```python
from build123d import *

# Parameters (mm, degrees)
F0_W     = 2140
F0_H     = 500
F1_DEPTH = 40
F2_W     = 600
F2_H     = 300
F3_DEPTH = 120
F5_D     = 45
F6_W     = 540
F6_H     = 240
F7_DEPTH = 120
F8_R     = 10
F10_D    = 45


with BuildPart() as f1:
    # F0 (on Top) → F1 (new body)
    with BuildSketch(Plane.XY):
        Rectangle(F0_W, F0_H)
    extrude(amount=F1_DEPTH)

    # F2 (on face) → F3 (join)
    with BuildSketch(Plane(origin=(0, 0, 0), x_dir=(1, 0, 0), z_dir=(0, 0, -1))):
        with Locations((-520, 0)):
            Rectangle(F2_W, F2_H)
    extrude(amount=F3_DEPTH)

    # F5 (through all)
    with Locations(Plane(origin=(0, 0, 0), x_dir=(1, 0, 0), z_dir=(0, 0, -1))):
        with Locations((-520, -200)):
            Hole(F5_D / 2)

    # F6 (on face) → F7 (cut)
    with BuildSketch(Plane.XY.offset(40)):
        with Locations((-520, 0)):
            Rectangle(F6_W, F6_H)
    extrude(amount=-F7_DEPTH, mode=Mode.SUBTRACT)

    # F8
    f8_edges = [f1.edges().sort_by_distance(p)[0] for p in [
        (-250, -120, -20),
        (-250, 0, -80),
        (-520, -120, -80),
        (-790, -120, -20),
        (-790, 0, -80),
        (-520, 120, -80),
        (-250, 120, -20),
        (-790, 120, -20),
    ]]
    fillet(f8_edges, radius=F8_R)

    # F10 (through all)
    with Locations(Plane.XY.offset(-80)):
        with Locations((-520, 0)):
            Hole(F10_D / 2)


solid = f1.part
```
Source: CAD feature listing. Evaluate the final solid. Frame: model axes, mm. A direction names the side the tool comes from. Give positions to 0.01 mm unless a question says otherwise; leave off trailing zeros. Order: outer loops, then holes, each group sorted by start corner. A loop starts at its lowest first (then second) coordinate and runs counter-clockwise, first axis right, second up. Notation, with made-up numbers: (-6.75, -20.5) -> (9.25, -20.5) arc R25 ccw to (9.25, 11.5) -> close; hole circle Ø5 at (-23, 48.25). An arc over 180 degrees is marked (long way). Use a Markdown table: item, result.
Q1. Section B-B (y = 0). Return the cut outline in (x, z).
A:
| item | result |
|---|---|
| outline | (-1070, 0) -> (-820, 0) -> (-820, -120) -> (-542.5, -120) -> (-542.5, -80) -> (-780, -80) arc R10 cw to (-790, -70) -> (-790, 40) -> (-1070, 40) -> close; (-497.5, -120) -> (-220, -120) -> (-220, 0) -> (1070, 0) -> (1070, 40) -> (-250, 40) -> (-250, -70) arc R10 cw to (-260, -80) -> (-497.5, -80) -> close |
Q2. First-contact query: P1, Ø1, axis at x = -662, z = -2.5, coming from the -Y side. Flat tip, straight axial feed; report the tip coordinate or a pass-through.
A:
| item | result |
|---|---|
| P1 | y = -150 |
Q3. Access query for faces 5 (the face through (-524, 26, -80)), 6 (the face through (-820, 2, -59)), 7 (the face through (-220, 2, -59)). Directions: +Z, -Z, +X, -X, +Y, -Y. A direction counts if a zero-diameter tool reaches every point of the face in a straight line with its end or side. Return the directions, or none.
A:
| item | result |
|---|---|
| face 5 | +Z |
| face 6 | -Z, -X, +Y, -Y |
| face 7 | -Z, +X, +Y, -Y |
Q4. Section C-C (z = -47.5). Return the cut outline in (x, y).
A:
| item | result |
|---|---|
| outline | (-820, -150) -> (-220, -150) -> (-220, 150) -> (-820, 150) -> close; hole (-790, -110) arc R10 ccw to (-780, -120) -> (-260, -120) arc R10 ccw to (-250, -110) -> (-250, 110) arc R10 ccw to (-260, 120) -> (-780, 120) arc R10 ccw to (-790, 110) -> close |
Q5. Material intervals for line 1 (Y direction, x = -520, z = 23); line 2 (Y direction, x = -764, z = 23); line 3 (Y direction, x = -520, z = -104), sorted ascending. Write a range as [from, to].
A:
| item | result |
|---|---|
| line 1 | [-250, -120], [120, 177.5], [222.5, 250] |
| line 2 | [-250, -120], [120, 250] |
| line 3 | [-150, -22.5], [22.5, 150] |
Q6. Section D-D (y = 200). Return the cut outline in (x, z), and give its area (3 significant figures).
A:
| item | result |
|---|---|
| outline | (-1070, 0) -> (-542.5, 0) -> (-542.5, 40) -> (-1070, 40) -> close; (-497.5, 0) -> (1070, 0) -> (1070, 40) -> (-497.5, 40) -> close |
| area | 83,800 mm^2 |
Q7. Section A-A (x = -520). Return the cut outline in (y, z).
A:
| item | result |
|---|---|
| outline | (-250, 0) -> (-150, 0) -> (-150, -120) -> (-22.5, -120) -> (-22.5, -80) -> (-110, -80) arc R10 cw to (-120, -70) -> (-120, 40) -> (-250, 40) -> close; (22.5, -120) -> (150, -120) -> (150, 0) -> (177.5, 0) -> (177.5, 40) -> (120, 40) -> (120, -70) arc R10 cw to (110, -80) -> (22.5, -80) -> close; (222.5, 0) -> (250, 0) -> (250, 40) -> (222.5, 40) -> close |
Q8. Pull-direction query (Y, two-part tool) for faces 1 (the face through (-524, 120, -14)), 2 (the face through (-524, 150, -59)), 3 (the face through (-541.46, 6.76, -100.28)), 4 (the face through (-524, -150, -59)); classes: +Y half, -Y half, draft (parallel to the pull), parting line (faces both ways), or undercut.
A:
| item | result |
|---|---|
| face 1 | undercut |
| face 2 | +Y half |
| face 3 | undercut |
| face 4 | -Y half |
